Here's how the part is built. I have some questions about the finished solid (model axes, mm). Give positions to 0.01 mm unless a question says otherwise; leave off trailing zeros. Write each loop counter-clockwise with the first axis right and the second up, starting at its lowest first coordinate (ties: lowest second). Pieces come first, ordered by that corner, then holes. Notation, with made-up numbers: (77, -38) -> (125, -38) arc R13 cw to (125, -24) -> close; hole circle Ø4 at (-33, 49). An arc over 180 degrees is marked (long way). Use CSV: the item, a comma, the result in double quotes. Start each with the question number.
(1) I need wall thicknesses on L1, parallel to X at y = 1.1, z = -7; L2, parallel to X at y = 4.05, z = -101; L3, parallel to X at y = 3.5, z = -118.5. Which ranges of each line are inside material? Lowest first, please. Write a range as [from, to].
(2) Suppose I cut it at A-A on x = -52.5. List the corners of the cut face in (y, z) for me.
(3) For pin 1 Ø9.5 at (x, z) = (-7, -7) entering from +Y; pin 2 Ø8 at (x, z) = (-27, -54.81) entering from -Y, each with a flat end and sliding along its axis, tell me the tip position at first contact or that it passes through.
(4) Suppose I cut it at D-D on z = -55. List the corners of the cut face in (x, y) for me, plus the area to 3 significant figures.
(5) Suppose I cut it at C-C on x = -97. List the corners of the cut face in (y, z) for me.
(6) Suppose I cut it at B-B on z = -7. List the corners of the cut face in (x, y) for me.
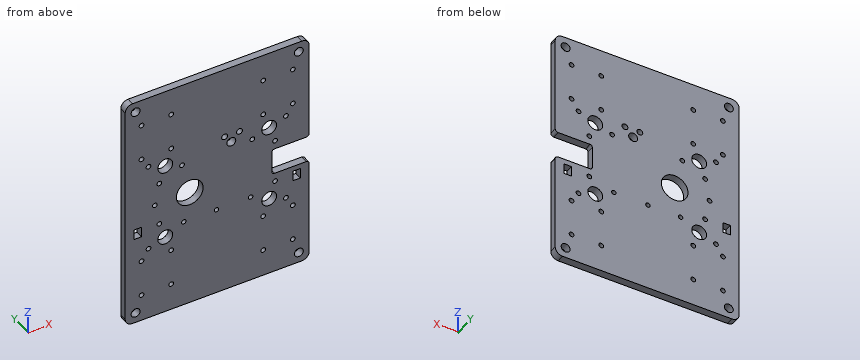
Autodesk Inventor part; units mm, degrees
ref_plane "YZ Plane" through (0, 0, 0) normal (1, 0, 0) x (0, 1, 0)
ref_plane "XZ Plane" through (0, 0, 0) normal (0, 1, 0) x (-1, 0, 0)
ref_plane "XY Plane" through (0, 0, 0) normal (0, 0, 1) x (1, 0, 0)
sketch "Sketch1" plane through (0, 0, 0) normal (0, 1, 0) x (-1, 0, 0)
  line L0 (0, 0) -> (124, 0)
  line L1 (124, 0) -> (124, -162)
  line L2 (124, -162) -> (0, -162)
  line L3 (0, -162) -> (0, 0)
  line L4 (117.9854, -81) -> (-11.1436, -81) construction
  line L5 (62, -11.2083) -> (62, -206.7638) construction
  circle A0 centre (113, -18.5) radius 1.6
  circle A1 centre (113, -43.5) radius 1.6
  circle A2 centre (93, -18.5) radius 1.6
  circle A3 centre (93, -43.5) radius 1.6
  circle A4 centre (113, -143.5) radius 1.6
  circle A5 centre (113, -118.5) radius 1.6
  circle A6 centre (93, -143.5) radius 1.6
  circle A7 centre (93, -118.5) radius 1.6
  circle A8 centre (11, -18.5) radius 1.6
  circle A9 centre (11, -43.5) radius 1.6
  circle A10 centre (31, -18.5) radius 1.6
  circle A11 centre (31, -43.5) radius 1.6
  circle A12 centre (11, -118.5) radius 1.6
  circle A13 centre (31, -143.5) radius 1.6
  circle A14 centre (11, -143.5) radius 1.6
  circle A15 centre (31, -118.5) radius 1.6
  line L6 (118, -93.5) -> (113, -93.5)
  line L7 (113, -93.5) -> (113, -100.5)
  line L8 (113, -100.5) -> (118, -100.5)
  line L9 (118, -100.5) -> (118, -93.5)
  line L10 (6, -93.5) -> (11, -93.5)
  line L11 (11, -93.5) -> (11, -100.5)
  line L12 (11, -100.5) -> (6, -100.5)
  line L13 (6, -100.5) -> (6, -93.5)
  circle A16 centre (7.5, -7.5) radius 2.8374
  circle A17 centre (37.5, -7.5) radius 2.5792
  circle A18 centre (7.5, -107.5) radius 2.9237
  circle A19 centre (37.5, -107.5) radius 2.6656
  dimension "d0" = 162
  dimension "d1" = 124
  dimension "d2" = 81
  dimension "d3" = 62
  dimension "d4" = 3.2
  dimension "d8" = 25
  dimension "d9" = 25
  dimension "d10" = 18.5
  dimension "d11" = 18.5
  dimension "d12" = 20
  dimension "d13" = 20
  dimension "d14" = 11
  dimension "d15" = 11
  dimension "d21" = 61.5
  dimension "d22" = 7
  dimension "d23" = 5
  dimension "d24" = 6
  dimension "d26" = 7.5
  dimension "d27" = 7.5
  dimension "d28" = 37.5
  dimension "d29" = 7.5
  dimension "d30" = 37.5
  dimension "d31" = 7.5
  dimension "d32" = 107.5
  dimension "d33" = 107.5
extrude "Extrusion1" add sketch "Sketch1" along normal blind 5 contours L0 L1 L2 L3 | A16 | A17 | A18 | A19
fillet "Fillet2" radius 5 4 edges at (0, 2.5, 0) (0, 2.5, -162) (-124, 2.5, -162) (-124, 2.5, 0)
sketch "Sketch3" plane through (0, 5, 0) normal (0, 1, 0) x (1, 0, 0)
  circle A0 centre (-93, 43.5) radius 3.1
  circle A1 centre (-93, 43.5) radius 1.8241
  line L0 (0, 5) -> (0, 157)
  circle A2 centre (-97, 54.8137) radius 4.621
  circle A3 centre (-97, 54.8137) radius 16
  line L1 (-112.1751, 81) -> (15.1489, 81) construction
  line L2 (-119, 0) -> (-5, 0)
  circle A4 centre (-93, 118.5) radius 3.1
  circle A5 centre (-93, 118.5) radius 1.8241
  circle A6 centre (-97, 107.1863) radius 4.621
  circle A7 centre (-97, 107.1863) radius 16
  circle A8 centre (-85.6863, 58.8137) radius 1.8241
  circle A9 centre (-101, 66.1274) radius 1.8241
  circle A10 centre (-108.3137, 50.8137) radius 1.8241
  circle A11 centre (-97, 54.8137) radius 4.621
  circle A12 centre (-101, 95.8726) radius 1.8241
  circle A13 centre (-108.3137, 111.1863) radius 1.8241
  line L3 (-124, 157) -> (-124, 5)
  line L4 (-62, -8.3299) -> (-62, 205.5694) construction
  circle A14 centre (-31, 43.5) radius 3.1
  circle A15 centre (-31, 43.5) radius 1.8241
  circle A16 centre (-27, 54.8137) radius 4.621
  circle A17 centre (-27, 54.8137) radius 16
  circle A18 centre (-31, 118.5) radius 3.1
  circle A19 centre (-31, 118.5) radius 1.8241
  circle A20 centre (-27, 107.1863) radius 4.621
  circle A21 centre (-27, 107.1863) radius 16
  circle A22 centre (-38.3137, 58.8137) radius 1.8241
  circle A23 centre (-23, 66.1274) radius 1.8241
  circle A24 centre (-15.6863, 50.8137) radius 1.8241
  circle A25 centre (-27, 54.8137) radius 4.621
  circle A26 centre (-15.6863, 111.1863) radius 1.8241
  circle A27 centre (-23, 95.8726) radius 1.8241
  circle A28 centre (-93, 43.5) radius 1.6
  point P0 (0, 0)
  dimension "d57" = 12
  dimension "d59" = 32
  dimension "d60" = 81
  dimension "d63" = 360
  dimension "d66" = 62
  dimension "d89" = 124
  dimension "d193" = 0
  dimension "d194" = 0
  dimension "d195" = 70
hole "Hole1" at (-108.3137, 5, -50.8137) at (-101, 5, -66.1274) at (-85.6863, 5, -58.8137) at (-108.3137, 5, -111.1863) at (-101, 5, -95.8726) at (-23, 5, -95.8726) at (-15.6863, 5, -111.1863) at (-38.3137, 5, -58.8137) at (-23, 5, -66.1274) at (-15.6863, 5, -50.8137) direction (0, -1, 0) diameter 3.2 end through all
sketch "Sketch4" plane through (0, 5, 0) normal (0, 1, 0) x (1, 0, 0)
  circle A0 centre (-97, 54.8137) radius 4
  circle A1 centre (-97, 107.1863) radius 4
  circle A2 centre (-27, 107.1863) radius 4
  circle A3 centre (-27, 54.8137) radius 4
  point P0 (0, 0)
  dimension "d196" = 70
hole "Hole2" at (-97, 5, -54.8137) at (-97, 5, -107.1863) at (-27, 5, -107.1863) at (-27, 5, -54.8137) direction (0, -1, 0) diameter 10 end through all
sketch "Sketch5" plane through (0, 5, 0) normal (0, 1, 0) x (1, 0, 0)
  circle A0 centre (-80.5, 81) radius 9
  line L0 (0, 5) -> (0, 157)
  line L1 (-119, 0) -> (-5, 0)
  circle A1 centre (-80.5, 81) radius 9 construction
  point P0 (0, 0)
  dimension "d81" = 18
  dimension "d82" = 80.5
  dimension "d83" = 81
  dimension "d90" = 18
extrude "Extrusion3" cut sketch "Sketch5" against normal blind 2
sketch "Sketch6" plane through (-80.5, 3, -81) normal (0, 1, 0) x (1, 0, 0)
  circle A0 centre (0, 0) radius 9
  point P0 (80.5, -81)
  dimension "d86" = 18
extrude "Extrusion4" cut sketch "Sketch6" against normal blind 3
sketch "Sketch7" plane through (0, 5, 0) normal (0, 1, 0) x (1, 0, 0)
  line L0 (-5, 162) -> (-119, 162)
  circle A0 centre (-84.5, 101) radius 1.5
  line L1 (-124, 157) -> (-124, 5)
  circle A1 centre (-62.5, 101) radius 1.5
  circle A2 centre (-39.5, 101) radius 1.5
  point P0 (0, 0)
  point P1 (-92.5, 103)
  point P2 (-47.5, 103)
  point P3 (-70.5, 103)
  dimension "d185" = 3
  dimension "d186" = 61
  dimension "d187" = 39.5
  dimension "d188" = 3
  dimension "d189" = 3
  dimension "d190" = 61.5
  dimension "d191" = 84.5
hole "Hole3" at (-84.5, 5, -101) at (-62.5, 5, -101) at (-39.5, 5, -101) direction (0, -1, 0) diameter 3 end through all
sketch "Sketch8" plane through (0, 5, 0) normal (0, 1, 0) x (1, 0, 0)
  line L0 (-147.8175, 81) -> (38.0677, 81) construction
  line L1 (-62, -18.8902) -> (-62, 202.7642) construction
  line L2 (-5, 162) -> (-119, 162)
  line L3 (-119, 0) -> (-5, 0)
  line L4 (0, 5) -> (0, 157)
  line L5 (-124, 157) -> (-124, 5)
  circle A0 centre (-7, 7) radius 3
  circle A1 centre (-7, 155) radius 3
  circle A2 centre (-117, 7) radius 3
  circle A3 centre (-117, 155) radius 3
  point P0 (0, 0)
  dimension "d104" = 162
  dimension "d105" = 124
  dimension "d106" = 62
  dimension "d107" = 81
  dimension "d108" = 6
  dimension "d109" = 7
  dimension "d110" = 7
hole "Hole4" at (-7, 5, -7) at (-117, 5, -7) at (-117, 5, -155) at (-7, 5, -155) direction (0, -1, 0) diameter 6 end through all
sketch "Sketch10" plane through (0, 5, 0) normal (0, 1, 0) x (1, 0, 0)
  line L0 (0, 5) -> (0, 157)
  line L1 (0, 72) -> (-25, 72)
  line L2 (-25, 72) -> (-25, 90)
  line L3 (-25, 90) -> (0, 90)
  line L4 (0, 90) -> (0, 72)
  line L5 (-119, 0) -> (-5, 0)
  point P0 (0, 0)
  point P1 (0, 90)
  dimension "d128" = 18
  dimension "d129" = 72
  dimension "d130" = 25
extrude "Extrusion5" cut sketch "Sketch10" against normal blind 10
fillet "Fillet4" radius 2 2 edges at (0, 2.5, -90) (0, 2.5, -72)
sketch "Sketch12" plane through (0, 0, 0) normal (0, -1, 0) x (1, 0, 0)
  circle A0 centre (-47, -49.5) radius 2
  circle A1 centre (-57, -49.5) radius 2
  line L0 (-119, 0) -> (-5, 0)
  line L1 (-40, -51) -> (-40, -46)
  circle A2 centre (-47, -49.5) radius 1.2295
  circle A3 centre (-47, -49.5) radius 1.2295
  circle A4 centre (-47, -49.5) radius 1.2295
  circle A5 centre (-57, -49.5) radius 1.2295
  point P0 (0, 0)
  dimension "d142" = 4
  dimension "d144" = 4
hole "Hole7" at (-47, 0, -49.5) at (-57, 0, -49.5) direction (0, 1, 0) diameter 4 depth 20 tip angle 118
sketch "Sketch13" plane through (0, 5, 0) normal (0, 1, 0) x (1, 0, 0)
  circle A0 centre (-104, 81) radius 1.5
  line L0 (-124, 157) -> (-124, 5)
  line L1 (-119, 0) -> (-5, 0)
  point P0 (0, 0)
  dimension "d154" = 3
  dimension "d155" = 20
  dimension "d156" = 81
hole "Hole8" at (-104, 5, -81) direction (0, -1, 0) diameter 3.2 depth 20 tip angle 118
sketch "Sketch14" plane through (0, 5, 0) normal (0, 1, 0) x (1, 0, 0)
  circle A0 centre (-52.5, 55) radius 3
  line L0 (-119, 0) -> (-5, 0)
  line L1 (0, 5) -> (0, 70)
  point P0 (0, 0)
  dimension "d164" = 55
  dimension "d165" = 52.5
  dimension "d166" = 6
hole "Hole9" at (-52.5, 5, -55) direction (0, -1, 0) diameter 6 depth 20 tip angle 118
fillet "Fillet6" radius 1.5 2 edges at (-25, 2.5, -72) (-25, 2.5, -90)
equation "\"d2\" = 0.5 * d0"
equation "\"d3\" = 0.5 * d1"
equation "\"d66\" = 0.5 * d89"
equation "\"d106\" = 0.5 * d105"
equation "\"d107\" = 0.5 * d104"
equation "\"d147\" = d144"
equation "\"d167\" = d166"
properties part number "x-Axis_plate_bottom_b" material "PET Plastic"
Geometry says:
1,L1,"[-124, -120], [-114, -10], [-4, 0]"
1,L2,"[-124, -86], [-83, -64], [-61, -41], [-38, 0]"
1,L3,"[-124, -114.6], [-111.4, -94.6], [-91.4, -32.6], [-29.4, -12.6], [-9.4, 0]"
2,outline,"(0, -162) -> (5, -162) -> (5, -58) -> (0, -58) -> close; (0, -52) -> (5, -52) -> (5, 0) -> (0, 0) -> close"
3,pin 1,"y = 5"
3,pin 2,"through"
4,outline,"(-124, 0) -> (-102, 0) -> (-102, 5) -> (-124, 5) -> close; (-92, 0) -> (-55.5, 0) -> (-55.5, 5) -> (-92, 5) -> close; (-49.5, 0) -> (-32, 0) -> (-32, 5) -> (-49.5, 5) -> close; (-22, 0) -> (0, 0) -> (0, 5) -> (-22, 5) -> close"
4,area,"490 mm²"
5,outline,"(0, -162) -> (5, -162) -> (5, -112.19) -> (0, -112.19) -> close; (0, -102.19) -> (5, -102.19) -> (5, -59.81) -> (0, -59.81) -> close; (0, -49.81) -> (5, -49.81) -> (5, 0) -> (0, 0) -> close"
6,outline,"(-124, 0) -> (-120, 0) -> (-120, 5) -> (-124, 5) -> close; (-114, 0) -> (-10, 0) -> (-10, 5) -> (-114, 5) -> close; (-4, 0) -> (0, 0) -> (0, 5) -> (-4, 5) -> close"
